Autodesk Inventor part; units mm, degrees
ref_plane "YZ Plane" through (0, 0, 0) normal (1, 0, 0) x (0, 1, 0)
ref_plane "XZ Plane" through (0, 0, 0) normal (0, 1, 0) x (-1, 0, 0)
ref_plane "XY Plane" through (0, 0, 0) normal (0, 0, 1) x (1, 0, 0)
sketch "Sketch1" plane through (0, 0, 0) normal (0, 0, 1) x (1, 0, 0)
  circle A0 centre (0, 0) radius 11
  dimension "d0" = 22
extrude "Extrusion1" add sketch "Sketch1" along normal blind 3.5
sketch "Sketch2" plane through (0, 0, 3.5) normal (0, 0, 1) x (1, 0, 0)
  circle A0 centre (0, 0) radius 5.1
  dimension "d3" = 10.2
extrude "Extrusion2" add sketch "Sketch2" along normal blind 10
sketch "Sketch3" plane through (0, 0, 3.5) normal (0, 0, 1) x (1, 0, 0)
  circle A0 centre (0, 0) radius 5.1
  point P0 (0, 8)
  dimension "d7" = 8
hole "Hole1" at (0, 8, 3.5) direction (0, 0, -1) diameter 3 depth 8 tip angle 118
pattern_circular "Circular Pattern1" count 4 over 360 about axis through (0, 0, 3.5) along (0, 0, 1) of "Hole1"
sketch "Sketch4" plane through (0, 0, 13.5) normal (0, 0, 1) x (1, 0, 0)
  circle A0 centre (0, 0) radius 4
  dimension "d18" = 8
extrude "Extrusion3" cut sketch "Sketch4" against normal through all
thread "Thread1"
properties part number "m8 nut"
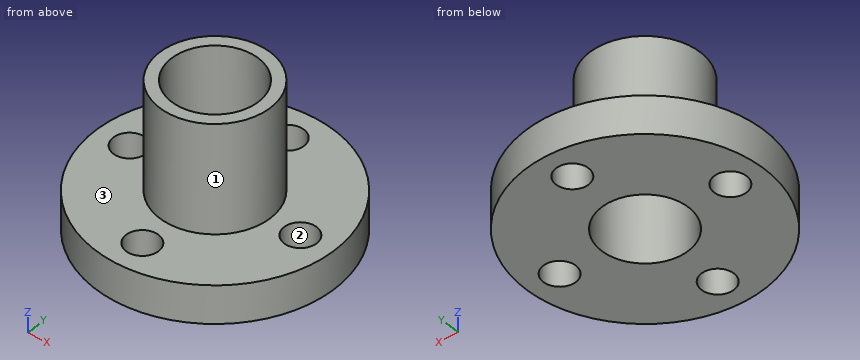
Verification items for the finished model (mm, model axes). Face numbers are marked on the shaded views. Round coordinates to 2 decimals unless told otherwise and drop trailing zeros. Write each loop counter-clockwise with the first axis right and the second up, starting at its lowest first coordinate (ties: lowest second). Pieces come first, ordered by that corner, then holes.
(1) Section check D-D (z = 1.5). Enter the section's corners in (x, y).
Returned:
outline: circle Ø22 at (0, 0); hole circle Ø3 at (-8, 0); hole circle Ø8 at (0, 0); hole circle Ø3 at (0, -8); hole circle Ø3 at (0, 8); hole circle Ø3 at (8, 0)
(2) Section check C-C (y = 3.5). Enter the section's corners in (x, z), plus the area to 3 significant figures.
Returned:
outline: (-10.43, 0) - (-1.94, 0) - (-1.94, 13.5) - (-3.71, 13.5) - (-3.71, 3.5) - (-10.43, 3.5) - close; (1.94, 0) - (10.43, 0) - (10.43, 3.5) - (3.71, 3.5) - (3.71, 13.5) - (1.94, 13.5) - close
area: 94.9 mm2
(3) Depth check by flat-ended pin: pin 1 Ø4 at (x, z) = (-0.5, 10.5) entering from -Y; pin 2 Ø1 at (y, z) = (-2.5, 6.5) entering from -X; pin 3 Ø3 at (x, y) = (-7, 5) entering from +Z. Enter the tip coordinate at first touch or a pass-through.
Returned:
pin 1: stops at y = -5.1
pin 2: stops at x = -4.69
pin 3: stops at z = 3.5
(4) Mould release check, pull along Y, two halves, no side actions. Record for the marked faces 1, 2 and 3: pulls with the +Y half, pulls with the -Y half, needs draft (parallel to the pull), parting line crosses it, or undercut.
Returned:
face 1: parting line crosses it
face 2: undercut
face 3: needs draft
(5) Material ranges on line 1 (Y direction, x = -8, z = 2.7); line 2 (Z direction, x = 1.75, y = -9.25); line 3 (Y direction, x = 0, z = 5.25), recorded low to high.
Returned:
line 1: y = -7.55 to -1.5, 1.5 to 7.55
line 2: z = 0 to 3.5
line 3: y = -5.1 to -4, 4 to 5.1
(6) Section check A-A (y = 0). Enter the section's corners in (x, z), plus the area to 3 significant figures.
Returned:
outline: (-11, 0) - (-9.5, 0) - (-9.5, 3.5) - (-11, 3.5) - close; (-6.5, 0) - (-4, 0) - (-4, 13.5) - (-5.1, 13.5) - (-5.1, 3.5) - (-6.5, 3.5) - close; (4, 0) - (6.5, 0) - (6.5, 3.5) - (5.1, 3.5) - (5.1, 13.5) - (4, 13.5) - close; (9.5, 0) - (11, 0) - (11, 3.5) - (9.5, 3.5) - close
area: 50.0 mm2
